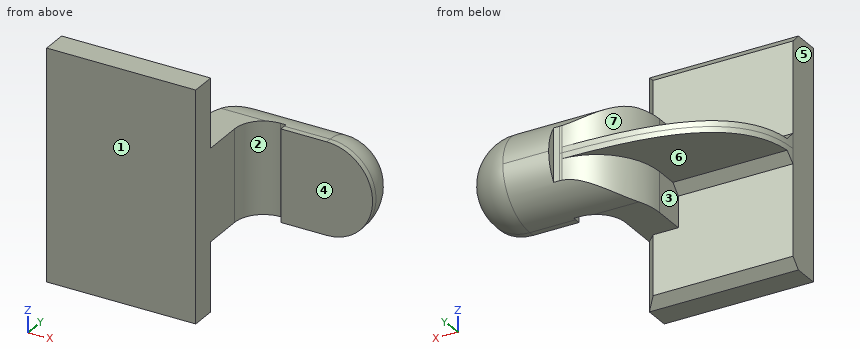
```python
from build123d import *

# Parameters (mm, degrees)
F1_DEPTH    = 63.5
F0_W        = 25.4
F0_H        = 19.05
F0_H_2      = 4.7752
F0_H_3      = 4.7498
F2_DEPTH    = 25.4
F3_DEPTH    = 3.175
F5_T1_DEPTH = 88.9
F5_T4_ANGLE = 180
F6_SIZE     = 5.08


# Not quite as in the source:
# - a fillet or chamfer that OpenCascade refuses, or shapes differently, is made with other operations: its cross-section is extruded or revolved along the edge and cut away or added


with BuildPart() as f1:
    # F0 (on Top) → F1 (new body, symmetric)
    with BuildSketch(Plane.XY):
        Polygon((41.275, -9.525), (41.275, 9.525), (22.225, 9.525), (-41.275, 9.525), (-41.275, -9.525), align=None)
    extrude(amount=F1_DEPTH, both=True)

    # F0 (on Top) → F2 (join, symmetric)
    with BuildSketch(Plane.XY):
        with BuildLine():
            Line((22.225, 9.525), (41.275, 9.525))
            Line((41.275, 9.525), (41.275, 27.0002))
            ThreePointArc((41.275, 27.0002), (45.9246798487, 38.2255201513), (57.15, 42.8752))
            Line((57.15, 42.8752), (60.325, 42.8752))
            Line((60.325, 42.8752), (60.325, 61.9252))
            Line((60.325, 61.9252), (57.15, 61.9252))
            add(Edge.make_bspline(
                [(55.7653482616, 61.897740953), (56.229278457, 61.90719099), (56.6908681229, 61.9163212607), (57.15, 61.9252)],
                knots=[110.2179933389, 110.2179933389, 110.2179933389, 110.2179933389, 111.5045361635, 111.5045361635, 111.5045361635, 111.5045361635], degree=3))
            ThreePointArc((55.7653482616, 61.897740953), (31.9695056943, 51.2014051666), (22.225, 27.0002))
            Line((22.225, 27.0002), (22.225, 9.525))
        make_face()
        with Locations((73.025, 52.4002)):
            Rectangle(F0_W, F0_H)
        with Locations((73.025, 40.4876)):
            Rectangle(F0_W, F0_H_2)
        with Locations((73.025, 64.3001)):
            Rectangle(F0_W, F0_H_3)
    extrude(amount=F2_DEPTH, both=True)

    # F0 (on Top) → F3 (join, symmetric)
    with BuildSketch(Plane.XY):
        with BuildLine():
            Line((-41.275, 9.525), (22.225, 9.525))
            Line((22.225, 9.525), (22.225, 27.0002))
            ThreePointArc((22.225, 27.0002), (31.9695056943, 51.2014051666), (55.7653482616, 61.897740953))
            add(Edge.make_bspline(
                [(-41.275, 9.525), (-40.9022788448, 57.9317022513), (16.0204954638, 61.0881572363), (55.7653482616, 61.897740953)],
                knots=[0, 0, 0, 0, 110.2179933389, 110.2179933389, 110.2179933389, 110.2179933389], degree=3))
        make_face()
    extrude(amount=F3_DEPTH, both=True)

    # F0 (on Top) → F4 (revolve)
    with BuildSketch(Plane.XY):
        Polygon((85.725, 61.9252), (85.725, 42.8752), (85.725, 38.1), (111.125, 38.1), (111.125, 66.675), (85.725, 66.675), align=None)
    revolve(axis=Axis((85.725, 52.3875, 0), (0, 1, 0)))

    # F5: fillet of radius 25.4 on 1 edges, made by hand

    # F5_s2 → F5_t1 (cut)
    with BuildSketch(Plane.YZ.offset(-3.175)):
        with BuildLine():
            ThreePointArc((66.675, 0), (59.2355122421, -17.9605122421), (41.275, -25.4))
            Line((41.275, -25.4), (66.675, -25.4))
            Line((66.675, -25.4), (66.675, 0))
        make_face()
        with BuildLine():
            ThreePointArc((66.675, 0), (59.2355122421, 17.9605122421), (41.275, 25.4))
            Line((41.275, 25.4), (66.675, 25.4))
            Line((66.675, 25.4), (66.675, 0))
        make_face()
    extrude(amount=F5_T1_DEPTH, mode=Mode.SUBTRACT)

    # F5_s3 → F5_t4 (revolve, cut)
    with BuildSketch(Plane.YZ.offset(85.725)):
        with BuildLine():
            ThreePointArc((66.675, 0), (59.2355122421, -17.9605122421), (41.275, -25.4))
            Line((41.275, -25.4), (66.675, -25.4))
            Line((66.675, -25.4), (66.675, 0))
        make_face()
    revolve(axis=Axis((85.725, 66.675, 0), (0, -1, 0)), revolution_arc=F5_T4_ANGLE, mode=Mode.SUBTRACT)

    # F6
    f6_edges = [f1.edges().sort_by_distance(p)[0] for p in [
        (-9.525, 9.525, 3.175),
        (-9.525, 9.525, -3.175),
        (0, 9.525, -63.5),
        (41.275, 9.525, -44.45),
        (41.275, 9.525, 44.45),
        (0, 9.525, 63.5),
    ]]
    chamfer(f6_edges, length=F6_SIZE)


solid = f1.part
```
Geometry check sheet. Reference: the model listing, model coordinates, mm. Face numbers are marked on the shaded views. A direction names the side the tool comes from. Coordinates: 2 decimals unless noted, no trailing zeros. Loops run counter-clockwise (first coordinate to the right, second up) from the corner with the lowest first, then second, coordinate; pieces in that order, holes last. Notation, with made-up numbers: (-22, 26.25) - (30, 26.25) arc R9 cw to (30, 36.25) - close; hole circle Ø7 at (4, -23.75). An arc over 180 degrees is marked (long way). One line per item, written item: value. Start each with the question number.
(1) Cross-section at B-B on z = -44. Enter the section's corners in (x, y) (3 decimals), plus the area to 3 significant figures.
(2) Cross-section at A-A on z = 21. Enter the section's corners in (x, y) (3 decimals).
(3) Depth check by flat-ended pin: P1, Ø14, axis at x = 40, y = 30, coming from the +Z side; P2, Ø1, axis at x = -7.5, z = 20.5, coming from the +Y side (3 decimals); P3, Ø10, axis at x = 11, y = 34.5, coming from the -Z side (3 decimals). Enter the tip coordinate at first touch or a pass-through.
(4) Tool access check on the marked faces 4, 5, 6 and 7. Record the directions out of +Z, -Z, +X, -X, +Y, -Y that give a thin tool (end or side, any length) a straight path to the whole face; none if there is none.
(5) Material ranges on line 1 (Y direction, x = 17.5, z = -44) (3 decimals); line 2 (Z direction, x = 23, y = 26); line 3 (Z direction, x = 14.5, y = 57.5) (3 decimals), recorded low to high. Write a range as [from, to].
(6) Mould release check, pull along X, two halves, no side actions. Record for the marked faces 1, 2 and 3: released by +X, released by -X, zero draft, split by the parting line, or undercut.
Results below:
1. outline: (-41.275, -9.525) - (41.275, -9.525) - (41.275, 4.445) - (36.195, 9.525) - (-41.275, 9.525) - close
1. area: 1,560 mm2
2. outline: (-41.275, -9.525) - (41.275, -9.525) - (41.275, 27) arc R15.875 cw to (57.15, 42.875) - (60.325, 42.875) - (60.325, 38.1) - (100.013, 38.1) - (100.013, 41.275) arc R14.288 ccw to (85.725, 55.563) - (37.053, 55.563) arc R34.925 ccw to (22.225, 27) - (22.225, 9.525) - (-41.275, 9.525) - close
3. P1: stops at z = 25.4
3. P2: stops at y = 9.525
3. P3: stops at z = -3.175
4. face 4: +Z, -Z, +X, -Y
4. face 5: +Z, -Z, -X, +Y, -Y
4. face 6: -Z, -X, +Y
4. face 7: +Z, -X, +Y
5. line 1: y = [-9.525, 9.525]
5. line 2: z = [-25.4, 25.4]
5. line 3: z = [-3.175, 3.175]
6. face 1: zero draft
6. face 2: undercut
6. face 3: released by -X
